Model file for the job. Use its own axes, mm. Face numbers are marked on the shaded views. A direction names the side the tool comes from. Coordinates: 2 decimals unless noted, no trailing zeros. Write each loop counter-clockwise with the first axis right and the second up, starting at its lowest first coordinate (ties: lowest second). Pieces come first, ordered by that corner, then holes. Notation, with made-up numbers: (37.25, 32.5) -> (73.25, 32.5) arc R15 ccw to (73.25, 48.5) -> close; hole circle Ø8 at (6, 82.25). An arc over 180 degrees is marked (long way). Answer as a JSON object with one key per item and string values. Group by question number.
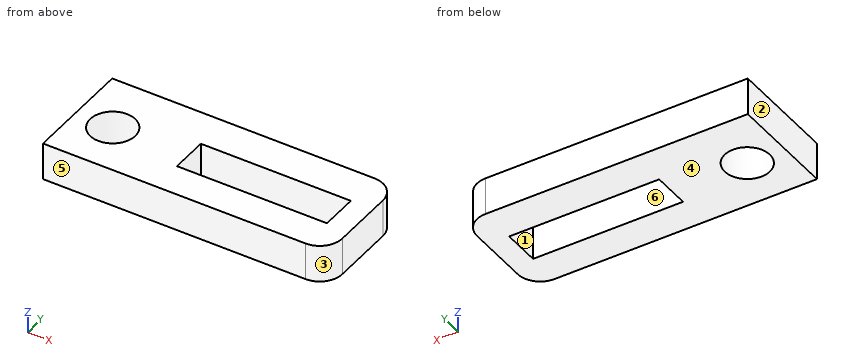
from build123d import *

# Parameters (mm, degrees)
SKETCH1_W           = 20
SKETCH1_H           = 5
BOSS_EXTRUDE1_DEPTH = 5


with BuildPart() as part:
    # Sketch1 → Boss-Extrude1 (new body)
    with BuildSketch(Plane.XY):
        with BuildLine():
            Line((77, 15), (42, 15))
            Line((42, 15), (42, 7.25))
            Line((42, 7.25), (42, 0.5))
            Line((42, 0.5), (77, 0.5))
            ThreePointArc((77, 0.5), (79.121320344, 1.378679656), (80, 3.5))
            Line((80, 3.5), (80, 12))
            ThreePointArc((80, 12), (79.121320344, 14.121320344), (77, 15))
        make_face()
        with BuildLine():
            ThreePointArc((50, 7.25), (47, 4.25), (44, 7.25))
            ThreePointArc((44, 7.25), (47, 10.25), (50, 7.25))
        make_face(mode=Mode.SUBTRACT)
        with Locations((67, 7.5)):
            Rectangle(SKETCH1_W, SKETCH1_H, mode=Mode.SUBTRACT)
    extrude(amount=BOSS_EXTRUDE1_DEPTH)


solid = part.part
(1) Cut at B-B on x = 47. List the corners of the cut face in (y, z), plus the area to 3 significant figures.
(2) Cut at C-C on z = 0.5. List the corners of the cut face in (x, y), plus the area to 3 significant figures.
(3) Cut at D-D on x = 66. List the corners of the cut face in (y, z).
(4) 3-axis set-ups, long thin cutter, end or side, ignore diameter. For the marked faces 5 and 6: which of +Z, -Z, +X, -X, +Y, -Y reach the whole face in a straight line?
(5) Cut at A-A on y = 7.25. List the corners of the cut face in (x, z), plus the area to 3 significant figures.
(6) Pull direction X, two halves, no side cores. Call the marked faces 1, 2, 3 and 4: released by +X, released by -X, zero draft, split by the parting line, or undercut.
(7) Wall check: probe 1 along X at (y, z) = (7.5, 2.95); probe 2 along Y at (x, z) = (62, 4.85); probe 3 along Y at (x, z) = (47, 2). Give the ranges that are in metal, low to high.
Results found:
{
 "1": {"outline": "(0.5, 0) -> (4.25, 0) -> (4.25, 5) -> (0.5, 5) -> close; (10.25, 0) -> (15, 0) -> (15, 5) -> (10.25, 5) -> close", "area": "42.5 mm²"},
 "2": {"outline": "(42, 0.5) -> (77, 0.5) arc R3 ccw to (80, 3.5) -> (80, 12) arc R3 ccw to (77, 15) -> (42, 15) -> close; hole circle Ø6 at (47, 7.25); hole (57, 5) -> (77, 5) -> (77, 10) -> (57, 10) -> close", "area": "419 mm²"},
 "3": {"outline": "(0.5, 0) -> (5, 0) -> (5, 5) -> (0.5, 5) -> close; (10, 0) -> (15, 0) -> (15, 5) -> (10, 5) -> close"},
 "4": {"face 5": "+Z, -Z, +X, -X, -Y", "face 6": "+Z, -Z"},
 "5": {"outline": "(42, 0) -> (44, 0) -> (44, 5) -> (42, 5) -> close; (50, 0) -> (57, 0) -> (57, 5) -> (50, 5) -> close; (77, 0) -> (80, 0) -> (80, 5) -> (77, 5) -> close", "area": "60.0 mm²"},
 "6": {"face 1": "undercut", "face 2": "released by -X", "face 3": "released by +X", "face 4": "zero draft"},
 "7": {"probe 1": "x = 42 to 44.01, 49.99 to 57, 77 to 80", "probe 2": "y = 0.5 to 5, 10 to 15", "probe 3": "y = 0.5 to 4.25, 10.25 to 15"}
}
